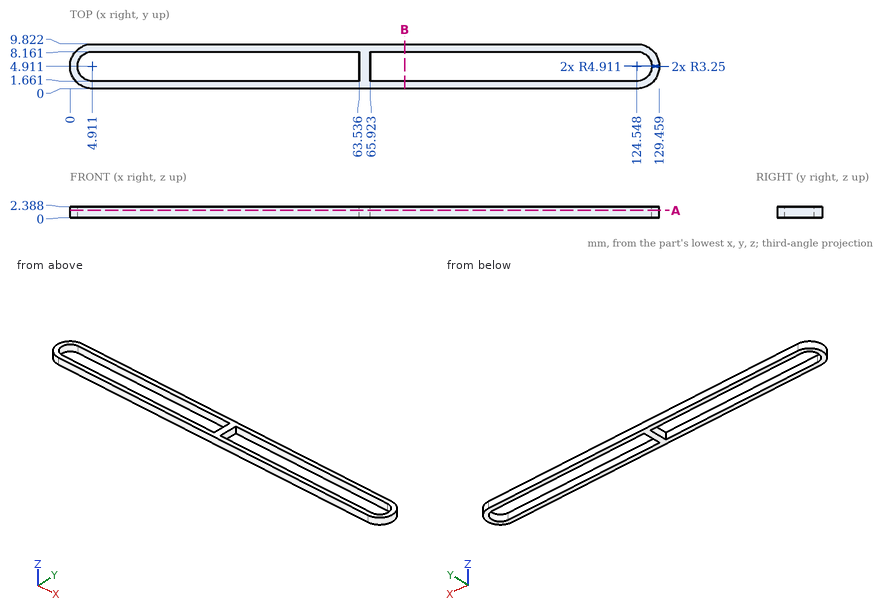
Input: dimensioned drawing with shaded views. Units: mm. Origin: part minimum x, y, z. Give positions to 0.01 mm unless a question says otherwise; leave off trailing zeros. Write each loop counter-clockwise with the first axis right and the second up, starting at its lowest first coordinate (ties: lowest second). Pieces come first, ordered by that corner, then holes. Notation, with made-up numbers: (-15, -36.5) -> (1, -36.5) arc R32 cw to (1, -3.5) -> close; hole circle Ø9 at (-11, 78.25). An arc over 180 degrees is marked (long way). Return JSON: item names as keys, results as strings. Group by question number.
1. Material intervals for line 1 (X direction, y = 4.5, z = 0.15) (1 decimal); line 2 (Y direction, x = 92, z = 1.25); line 3 (X direction, y = 7, z = 2.15) (1 decimal), sorted ascending. Write a range as from..to.
2. Section B-B, the plane x = 73.5. Output: boundary loops of the cut face in (y, z).
3. Section A-A, the plane z = 1.6. Count the separate pieces of the cut face and the enclosed holes in it.
Determined:
{
 "1": {"line 1": "x = 0..1.7, 63.5..65.9, 127.8..129.4", "line 2": "y = 0..1.66, 8.16..9.82", "line 3": "x = 0.5..2.4, 63.5..65.9, 127..129"},
 "2": {"outline": "(0, 0) -> (1.66, 0) -> (1.66, 2.39) -> (0, 2.39) -> close; (8.16, 0) -> (9.82, 0) -> (9.82, 2.39) -> (8.16, 2.39) -> close"},
 "3": {"separate pieces": "1", "enclosed holes": "2"}
}
